from build123d import *

# Parameters (mm, degrees)
SKETCH2_W           = 80
SKETCH2_H           = 10
BOSS_EXTRUDE1_DEPTH = 0.5
SKETCH3_R           = 2.65
SKETCH3_R_2         = 2.6
SKETCH3_R_3         = 2.55
SKETCH3_R_4         = 2.5
BOSS_EXTRUDE2_DEPTH = 5
FILLET1_R           = 1
FILLET2_R           = 10


with BuildPart() as part:
    # Sketch2 → Boss-Extrude1 (new body)
    with BuildSketch(Plane(origin=(0, 0, 0), x_dir=(1, 0, 0), z_dir=(0, 1, 0))):
        Rectangle(SKETCH2_W, SKETCH2_H)
    extrude(amount=BOSS_EXTRUDE1_DEPTH)

    # Sketch3 → Boss-Extrude2 (add)
    with BuildSketch(Plane(origin=(0, 0.5, 0), x_dir=(1, 0, 0), z_dir=(0, 1, 0))):
        with Locations(Location((-30, 0, 0), (0, 0, 270))):
            Circle(SKETCH3_R)
        with Locations(Location((-10, 0, 0), (0, 0, 270))):
            Circle(SKETCH3_R_2)
        with Locations(Location((10, 0, 0), (0, 0, 270))):
            Circle(SKETCH3_R_3)
        with Locations(Location((30, 0, 0), (0, 0, 270))):
            Circle(SKETCH3_R_4)
    extrude(amount=BOSS_EXTRUDE2_DEPTH)

    # Fillet1
    fillet1_edges = [part.edges().sort_by_distance(p)[0] for p in [
        (-30, 5.5, -2.65),
        (-10, 5.5, -2.6),
        (10, 5.5, -2.55),
        (30, 5.5, -2.5),
    ]]
    fillet(fillet1_edges, radius=FILLET1_R)

    # Fillet2
    # the kernel refuses this fillet: 10 mm, written as the material it takes off along each edge
    with BuildSketch(Plane(origin=(-40, -25, -5), x_dir=(1, 0, 0), z_dir=(0, 1, 0)), Plane(origin=(-40, -25, 5), x_dir=(0, 0, -1), z_dir=(0, 1, 0))) as fillet2_piece_1:
        with BuildLine():
            CenterArc((FILLET2_R, -FILLET2_R), FILLET2_R, 90, 90)
            Line((0, -FILLET2_R), (0, 0))
            Line((0, 0), (FILLET2_R, 0))
        make_face()
    extrude(amount=50.5, mode=Mode.SUBTRACT)


solid = part.part
Geometry: final body of the model. Coordinates: model frame, mm. A direction names the side the tool comes from. Round coordinates to 2 decimals unless told otherwise and drop trailing zeros. Loops run counter-clockwise (first coordinate to the right, second up) from the corner with the lowest first, then second, coordinate; pieces in that order, holes last. Notation, with made-up numbers: M 4,40 L 13,40 A28 cw 13,59 Z; hole C 79,52.25 d5. An arc over 180 degrees is marked long. Put each result on its own line as item: value. Start each with the question number.
(1) Section query B-B (y = 1.4). Return loops of the section in (x, z), then the cut area to 3 significant figures.
(2) Draft query along X for faces 3 (the face through (32.11, 2.47, 1.34)), 4 (the face through (-30, 5.5, 0)), 5 (the face through (-34.936, 0.247, -3.697)). Return one class per face: +X half, -X half, draft (parallel to the pull), parting line (faces both ways), or undercut.
(3) Material intervals for line 1 along X through (y, z) = (4.4, 2); line 2 along X through (y, z) = (0.7, 1.5); line 3 along Y through (x, z) = (27.5, 3.5), sorted ascending. Write a range as [from, to].
(4) Section query A-A (x = 30). Return loops of the section in (y, z), then the cut area to 3 significant figures.
(5) Section query C-C (x = -10). Return loops of the section in (y, z).
(6) Section query D-D (x = 17). Return loops of the section in (y, z), then the cut area to 3 significant figures.
(7) Contact query for flat-ended pins moving along their axis: pin 1 Ø6 at (x, z) = (11.5, -3) entering from -Y; pin 2 Ø1.5 at (x, z) = (18, -1.5) entering from +Y. Output: stop coordinate, or through.
(8) Set-up query: faces 1 (the face through (7.51, 2.47, -0.55)), 2 (the face through (-10, 5.5, 0)). Return all of +Z, -Z, +X, -X, +Y, -Y with unobstructed straight access to the full face (end or side cutting, diameter ignored); none if empty.
Findings below:
1. outline: C -30,0 d5.3; C -10,0 d5.2; C 10,0 d5.1; C 30,0 d5
1. area: 83.4 mm2
2. face 3: undercut
2. face 4: draft
2. face 5: -X half
3. line 1: x = [-31.74, -28.26], [-11.66, -8.34], [8.42, 11.58], [28.5, 31.5]
3. line 2: x = [-32.18, -27.82], [-12.12, -7.88], [7.94, 12.06], [28, 32]
3. line 3: y = [0, 0.5]
4. outline: M 0,-5 L 0.5,-5 L 0.5,-2.5 L 4.5,-2.5 A1 ccw 5.5,-1.5 L 5.5,1.5 A1 ccw 4.5,2.5 L 0.5,2.5 L 0.5,5 L 0,5 Z
4. area: 29.6 mm2
5. outline: M 0,-5 L 0.5,-5 L 0.5,-2.6 L 4.5,-2.6 A1 ccw 5.5,-1.6 L 5.5,1.6 A1 ccw 4.5,2.6 L 0.5,2.6 L 0.5,5 L 0,5 Z
6. outline: M 0,-5 L 0.5,-5 L 0.5,5 L 0,5 Z
6. area: 5.00 mm2
7. pin 1: stops at y = 0
7. pin 2: stops at y = 0.5
8. face 1: +Y
8. face 2: +Z, -Z, +X, -X, +Y
